Read the model definition and answer for the solid it produces. Units are mm, in the model's axes. Face numbers are marked on the shaded views. Coordinates: 2 decimals unless noted, no trailing zeros. Write each loop counter-clockwise with the first axis right and the second up, starting at its lowest first coordinate (ties: lowest second). Pieces come first, ordered by that corner, then holes.
Item 1: Section B-B (z = -13) is taken. Give the vertices of the cut face in (x, y).
Item 2: Determine the mould class of the marked faces 1, 2 and 3 for opening direction X: released by +X, released by -X, zero draft, split by the parting line, or undercut.
Item 3: Straight lines are drawn through the part: probe 1 along Y at (x, z) = (17.5, 29); probe 2 along Y at (x, z) = (288.5, -37); probe 3 along Z at (x, y) = (29.5, 7.5). For each, find the intervals that lie inside material, in ascending order.
Item 4: Each of these flat-tipped pins is pushed along its axis until it touches: P1, Ø3, axis at x = 84, y = 0, coming from the +Z side; P2, Ø1.8, axis at x = 154.5, y = -17.5, coming from the -Z side; P3, Ø6, axis at x = 63, z = 31.5, coming from the +Y side. Where does it stop, or does it pass through?
Item 5: Section A-A (x = 224) is taken. Give the vertices of the cut face in (y, z).
from build123d import *

# Parameters (mm, degrees)
F0_W     = 10.2
F0_H     = 75
F1_DEPTH = 300
F2_W     = 290
F2_H     = 70
F3_DEPTH = 5
F4_W     = 290
F4_H     = 10.2
F5_DEPTH = 80
F6_SIZE  = 1.5


# Not quite as in the source:
# - a feature names something its author has since deleted; it is built from what else it names


with BuildPart() as f1:
    # F0 (on Right) → F1 (new body)
    with BuildSketch(Plane.YZ):
        Polygon((-10.1, -42.5), (10.1, -42.5), (10.1, 42.5), (-27.6, 42.5), (-27.6, 27.5), (-22.6, 27.5), (-22.6, 33.5), (-22.6, 37.5), (-18.6, 37.5), (-15.1, 37.5), (-10.1, 37.5), (-10.1, 32.5), align=None)
        Rectangle(F0_W, F0_H, mode=Mode.SUBTRACT)
        with BuildLine():
            ThreePointArc((-22.6, 33.5), (-21.4284271247, 36.3284271247), (-18.6, 37.5))
            Line((-18.6, 37.5), (-22.6, 37.5))
            Line((-22.6, 37.5), (-22.6, 33.5))
        make_face()
        with BuildLine():
            ThreePointArc((-15.1, 37.5), (-11.5644660941, 36.0355339059), (-10.1, 32.5))
            Line((-10.1, 32.5), (-10.1, 37.5))
            Line((-10.1, 37.5), (-15.1, 37.5))
        make_face()
        Rectangle(F0_W, F0_H)
    extrude(amount=F1_DEPTH)

    # F2 (on face) → F3 (cut)
    with BuildSketch(Plane(origin=(0, 10.1, 0), x_dir=(-1, 0, 0), z_dir=(0, 1, 0))):
        with Locations((-150, 2.5)):
            Rectangle(F2_W, F2_H)
    extrude(amount=-F3_DEPTH, mode=Mode.SUBTRACT)

    # F4 (on face) → F5 (cut)
    with BuildSketch(Plane.XY.offset(42.5)):
        with Locations((150, 0)):
            Rectangle(F4_W, F4_H)
    extrude(amount=-F5_DEPTH, mode=Mode.SUBTRACT)

    # F6
    f6_edges = [f1.edges().sort_by_distance(p)[0] for p in [
        (300, 0, -42.5),
        (300, 10.1, 0),
        (300, -8.75, 42.5),
        (300, -27.6, 35),
        (300, -25.1, 27.5),
        (300, -22.6, 30.5),
        (300, -21.428427, 36.328427),
        (300, -16.85, 37.5),
        (300, -11.564466, 36.035534),
        (300, -10.1, -5),
        (150, 10.1, -42.5),
        (0, 10.1, 0),
        (150, 10.1, 42.5),
        (5, 10.1, 2.5),
        (150, 10.1, -32.5),
        (295, 10.1, 2.5),
        (150, 10.1, 37.5),
        (0, -8.75, 42.5),
        (150, -27.6, 42.5),
        (150, -5.1, 42.5),
        (5, 0, 42.5),
        (150, 5.1, 42.5),
        (295, 0, 42.5),
        (150, -10.1, -42.5),
        (0, 0, -42.5),
        (0, -27.6, 35),
        (0, -25.1, 27.5),
        (0, -22.6, 30.5),
        (0, -21.428427, 36.328427),
        (0, -16.85, 37.5),
        (0, -11.564466, 36.035534),
        (0, -10.1, -5),
    ]]
    chamfer(f6_edges, length=F6_SIZE)


solid = f1.part
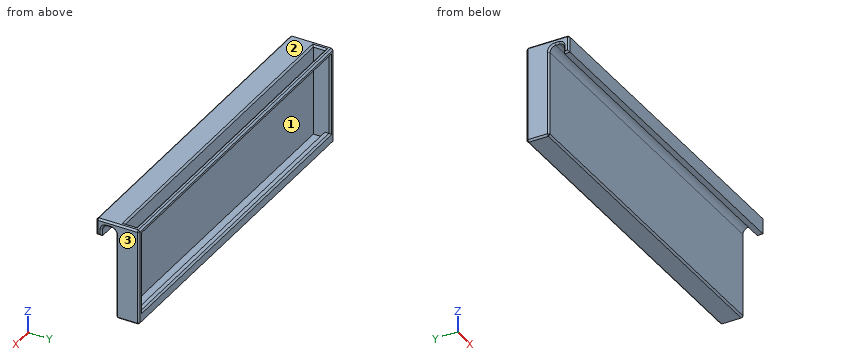
Established:
1. outline: (0, -8.6) - (1.5, -10.1) - (298.5, -10.1) - (300, -8.6) - (300, 8.6) - (298.5, 10.1) - (296.5, 10.1) - (295, 8.6) - (295, -5.1) - (5, -5.1) - (5, 8.6) - (3.5, 10.1) - (1.5, 10.1) - (0, 8.6) - close
2. face 1: undercut
2. face 2: zero draft
2. face 3: released by +X
3. probe 1: y = -27.6 to -22.6, -10.1 to -5.1
3. probe 2: y = -10.1 to -5.1, 5.1 to 10.1
3. probe 3: z = -42.5 to -32.5, 37.5 to 42.5
4. P1: stops at z = -37.5
4. P2: stops at z = 37.5
4. P3: stops at y = -5.1
5. outline: (-27.6, 27.5) - (-22.6, 27.5) - (-22.6, 33.5) arc R4 cw to (-18.6, 37.5) - (-15.1, 37.5) arc R5 cw to (-10.1, 32.5) - (-10.1, -41) - (-8.6, -42.5) - (8.6, -42.5) - (10.1, -41) - (10.1, -34) - (8.6, -32.5) - (5.1, -32.5) - (5.1, -37.5) - (-5.1, -37.5) - (-5.1, 41) - (-6.6, 42.5) - (-26.1, 42.5) - (-27.6, 41) - close; (5.1, 37.5) - (8.6, 37.5) - (10.1, 39) - (10.1, 41) - (8.6, 42.5) - (6.6, 42.5) - (5.1, 41) - close
